Solid Edge part; units mm, degrees
sketch "Sketch1" plane through (0, 0, 0) normal (0, 0, 1) x (1, 0, 0)
  line L0 (-70, 70) -> (70, 70)
  line L1 (70, 70) -> (70, -70)
  line L2 (70, -70) -> (-70, -70)
  line L3 (-70, -70) -> (-70, 70)
  dimension "D1" = 70
  dimension "D2" = 70
extrude "Protrusion1" add sketch "Sketch1" along normal blind 15
hole "Hole_1" at (38.8909, 38.8909, 15) direction (0, 0, -1) diameter 4.917 end up to next thread major 6 thread length 2
hole "Hole1" at (38.8909, -38.8909, 15) direction (0, 0, -1) diameter 4.917 end up to next thread major 6 thread length 2
hole "Hole2" at (-38.8909, -38.8909, 15) direction (0, 0, -1) diameter 4.917 end up to next thread major 6 thread length 2
hole "Hole3" at (-38.8909, 38.8909, 15) direction (0, 0, -1) diameter 4.917 end up to next thread major 6 thread length 2
hole "Hole_5" at (50, 50, 15) direction (0, 0, -1) diameter 9 end up to next counterbore diameter 15 counterbore depth 8.8
hole "Hole4" at (-50, 50, 15) direction (0, 0, -1) diameter 9 end up to next counterbore diameter 15 counterbore depth 8.8
hole "Hole5" at (-50, -50, 15) direction (0, 0, -1) diameter 9 end up to next counterbore diameter 15 counterbore depth 8.8
hole "Hole6" at (50, -50, 15) direction (0, 0, -1) diameter 9 end up to next counterbore diameter 15 counterbore depth 8.8
hole "Hole_9" at (55, -10, 15) direction (0, 0, -1) diameter 5 end up to next
hole "Hole7" at (-55, -10, 15) direction (0, 0, -1) diameter 5 end up to next
fillet "Round_1" radius 15 4 edges at (-70, 70, 7.5) (70, -70, 7.5) (-70, -70, 7.5) (70, 70, 7.5)
chamfer "Chamfer_2" distance 2 angle 45 7 edges at (-70, 0, 15) (0, 70, 15) (65.6066, 65.6066, 15) (70, 0, 15) (65.6066, -65.6066, 15) (0, -70, 15) (-65.6066, -65.6066, 15)
The model under review builds one solid part; all positions refer to its coordinate system, in mm. A direction names the side the tool comes from. Coordinates: 2 decimals unless noted, no trailing zeros. Write each loop counter-clockwise with the first axis right and the second up, starting at its lowest first coordinate (ties: lowest second). Pieces come first, ordered by that corner, then holes. Notation, with made-up numbers: (57, 87) - (83, 87) arc R23 cw to (83, 107) - close; hole circle Ø2 at (-2, 56). An arc over 180 degrees is marked (long way). Answer as a JSON object with one key per item and string values. Group by question number.
1. Add section B-B (x = -50). Give the boundary of the cut face in (y, z).
2. Clearance check with a flat-ended pin moving along its axis: pin 1 Ø7.5 at (x, y) = (47, -51) entering from +Z. State where the tip first meets the part, or that it passes through.
3. Add section C-C (z = 3.5). Give the number of separate pieces and of enclosed holes in the cut face, plus the area to 3 significant figures.
4. Machinability: for faces 4 (the face through (-40.39, -36.94, 7.6)), 5 (the face through (57.32, -48.37, 10.54)), which of the approach directions +Z, -Z, +X, -X, +Y, -Y give a long, thin tool a straight path to every point of the face, cutting with its end or side? Answer none if there is none.
5. Mouldability with a two-part tool opening along Y and no side actions: class faces 1 (the face through (57.32, 51.63, 10.54)), 2 (the face through (1, 1, 15)), 3 (the face through (1, -70, 6)) as pulls with the +Y half, pulls with the -Y half, needs draft (parallel to the pull), parting line crosses it, or undercut.
6. Add section A-A (y = -10). Give the boundary of the cut face in (x, z), plus the area to 3 significant figures.
7. To check wall thickness, follow probe 1 along X at (y, z) = (-10, 5.5); probe 2 along Y at (x, z) = (-50, 9.5); probe 3 along Y at (x, z) = (-38.5, 11.75). State the ranges of each line that lie inside material, in increasing order.
Findings:
{
 "1": {"outline": "(-70, 0) - (-54.5, 0) - (-54.5, 6.2) - (-57.5, 6.2) - (-57.5, 15) - (-68, 15) - (-70, 13) - close; (-45.5, 0) - (45.5, 0) - (45.5, 6.2) - (42.5, 6.2) - (42.5, 15) - (-42.5, 15) - (-42.5, 6.2) - (-45.5, 6.2) - close; (54.5, 0) - (70, 0) - (70, 13) - (68, 15) - (57.5, 15) - (57.5, 6.2) - (54.5, 6.2) - close"},
 "2": {"pin 1": "z = 6.2"},
 "3": {"separate pieces": "1", "enclosed holes": "10", "area": "19,000 mm²"},
 "4": {"face 4": "+Z, -Z", "face 5": "+Z"},
 "5": {"face 1": "undercut", "face 2": "needs draft", "face 3": "pulls with the -Y half"},
 "6": {"outline": "(-70, 0) - (-57.5, 0) - (-57.5, 15) - (-68, 15) - (-70, 13) - close; (-52.5, 0) - (52.5, 0) - (52.5, 15) - (-52.5, 15) - close; (57.5, 0) - (70, 0) - (70, 13) - (68, 15) - (57.5, 15) - close", "area": "1,950 mm²"},
 "7": {"probe 1": "-70 to -57.5, -52.5 to 52.5, 57.5 to 70", "probe 2": "-70 to -57.5, -42.5 to 42.5, 57.5 to 70", "probe 3": "-70 to -41.32, -36.46 to 36.46, 41.32 to 70"}
}
